Autodesk Inventor part; units mm, degrees
ref_plane "YZ Plane" through (0, 0, 0) normal (1, 0, 0) x (0, 1, 0)
ref_plane "XZ Plane" through (0, 0, 0) normal (0, 1, 0) x (-1, 0, 0)
ref_plane "XY Plane" through (0, 0, 0) normal (0, 0, 1) x (1, 0, 0)
sketch "Part" plane through (0, 0, 0) normal (1, 0, 0) x (0, 1, 0)
  line L0 (-0.5368, 0.0583) -> (59.7882, 0.0583) construction
  line L1 (-0.5371, -0.7417) -> (44.8022, -0.7417) construction
  arc A0 (59.7829, -0.7417) -> (59.7882, 0.0583) centre (-0.5368, 0.0583) ccw construction
  line L2 (-0.5368, 0.0583) -> (49.9741, -29.1042) construction
  arc A1 (47.3067, -27.5642) -> (54.7024, -0.7417) centre (-0.5368, 0.0583) ccw construction
  line L3 (69.9104, -5.8217) -> (54.3944, -5.8217) construction
  arc A2 (51.7936, -29.9522) -> (59.7829, -0.7417) centre (-0.5368, 0.0583) ccw construction
  line L4 (-0.5368, 0.0583) -> (66.9803, -116.8847) construction
  arc A3 (29.6257, -52.1846) -> (51.7936, -29.9522) centre (-0.5368, 0.0583) ccw
  arc A4 (27.0857, -47.7852) -> (54.3944, -5.8217) centre (-0.5368, 0.0583) ccw
  arc A5 (54.7024, -0.7417) -> (54.7082, 0.0583) centre (-0.5368, 0.0583) ccw construction
  line L5 (54.7024, -0.7417) -> (59.7829, -0.7417) construction
  line L6 (57.491, -5.8217) -> (54.3944, -5.8217) construction
  line L7 (44.8022, 0.0583) -> (44.8022, -0.7417) construction
  line L8 (44.8022, -0.7417) -> (44.8022, -5.8217)
  line L9 (44.8022, -5.8217) -> (44.8022, -11.0315) construction
  line L10 (44.8022, -0.7417) -> (57.7827, -0.7417)
  line L11 (44.8022, -5.8217) -> (-19.8971, -5.8217) construction
  line L12 (49.2882, 5.599) -> (49.2882, -56.7812) construction
  arc A6 (28.6257, -50.4526) -> (49.9741, -29.1042) centre (-0.5368, 0.0583) ccw construction
  line L13 (54.3944, -5.8217) -> (50.4651, -5.8217) construction
  line L14 (54.3944, -5.8217) -> (44.8022, -5.8217)
  line L15 (49.9741, -29.1042) -> (51.7936, -29.9522)
  arc A7 (49.9741, -29.1042) -> (57.7827, -0.7417) centre (-0.5368, 0.0583) ccw
  arc A8 (57.7827, -0.7417) -> (57.7882, 0.0583) centre (-0.5368, 0.0583) ccw construction
  line L16 (-0.5368, 0.0583) -> (-30.6993, -52.1846) construction
  line L17 (0.1561, -0.3414) -> (-22.5135, -39.6064) construction
  arc A9 (-30.6993, -52.1846) -> (-30.0039, -52.5801) centre (-0.5368, 0.0583) ccw construction
  line L18 (-0.5368, 0.0583) -> (-0.5368, -58.2667) construction
  arc A10 (-27.4636, -48.1802) -> (-0.5368, -55.1867) centre (-0.5368, 0.0583) ccw construction
  line L19 (-30.6682, -63.8907) -> (-22.9102, -50.4535) construction
  arc A11 (-30.0039, -52.5801) -> (-0.7122, -60.2664) centre (-0.5368, 0.0583) ccw construction
  arc A12 (-0.7122, -60.2664) -> (29.6257, -52.1846) centre (-0.5368, 0.0583) ccw
  arc A13 (-22.9102, -50.4535) -> (27.0857, -47.7852) centre (-0.5368, 0.0583) ccw
  arc A14 (-28.1593, -47.7852) -> (-27.4636, -48.1802) centre (-0.5368, 0.0583) ccw construction
  line L20 (-27.4636, -48.1802) -> (-30.0039, -52.5801) construction
  line L21 (-24.4585, -53.1353) -> (-22.9102, -50.4535) construction
  line L22 (-23.2063, -39.2064) -> (-22.5135, -39.6064) construction
  line L23 (-22.5135, -39.6064) -> (-18.1141, -42.1464)
  line L24 (-18.1141, -42.1464) -> (-13.6022, -44.7513) construction
  line L25 (-22.5135, -39.6064) -> (-29.0038, -50.8478)
  line L26 (-18.1141, -42.1464) -> (14.2355, 13.8848) construction
  line L27 (-30.2477, -40.3211) -> (23.7751, -71.5111) construction
  arc A15 (-0.5368, -58.2667) -> (28.6257, -50.4526) centre (-0.5368, 0.0583) ccw construction
  line L28 (-22.9102, -50.4535) -> (-20.9456, -47.0506) construction
  line L29 (-22.9102, -50.4535) -> (-18.1141, -42.1464)
  line L30 (-0.5368, -58.2667) -> (-0.7122, -60.2664)
  arc A16 (-29.0038, -50.8478) -> (-0.5368, -58.2667) centre (-0.5368, 0.0583) ccw
  arc A17 (-29.6993, -50.4526) -> (-29.0038, -50.8478) centre (-0.5368, 0.0583) ccw construction
  dimension "d29" = 60.325
  dimension "d32" = 30
  dimension "d35" = 5.08
  dimension "d37" = 60
  dimension "d38" = 55.245
  dimension "d42" = 14.986
  dimension "d44" = 10.5
  dimension "d45" = 58.325
  dimension "d64" = 0.8
extrude "Extrusion2" add sketch "Part" along normal blind 5.08
sketch "Sketch5" plane through (0, 44.8022, -0.7417) normal (0, 0, 1) x (1, 0, 0)
  line L0 (0, 12.9805) -> (5.08, 12.9805)
  line L1 (2.54, 12.9805) -> (2.54, 0) construction
  line L2 (0, 0) -> (5.08, 0)
  line L3 (0, 4.4805) -> (5.08, 4.4805) construction
  point P0 (0, -44.8022)
  point P1 (2.54, 4.4805)
  dimension "d48" = 8.5
hole "Hole1" at (2.54, 49.2827, -0.7417) direction (0, 0, -1) diameter 2.4384 depth 12.2936 tip angle 118
sketch "Sketch6" plane through (0, -29.0038, -50.8478) normal (0, -0.866, 0.5) x (1, 0, 0)
  line L0 (0, 12.9805) -> (5.08, 12.9805) construction
  line L1 (2.54, 12.9805) -> (2.54, 0) construction
  line L2 (0, 0) -> (5.08, 0) construction
  line L3 (0, 5.9891) -> (0, 58.4948) construction
  line L4 (0, 8.5) -> (5.08, 8.5) construction
  line L5 (5.08, 5.9891) -> (5.08, 58.4948) construction
  point P0 (0, 58.5374)
  point P1 (2.54, 8.5)
  dimension "d56" = 8.5
hole "Hole2" at (2.54, -24.7538, -43.4866) direction (0, 0.866, -0.5) diameter 2.4384 depth 12.2936 tip angle 118
equation "\"d35\" = d29 - d34"
properties part number "new_insert"
Geometry check sheet. Reference: the model listing, model coordinates, mm. A direction names the side the tool comes from. Round coordinates to 2 decimals unless told otherwise and drop trailing zeros. Loops run counter-clockwise (first coordinate to the right, second up) from the corner with the lowest first, then second, coordinate; pieces in that order, holes last. Notation, with made-up numbers: (19, 89.5) - (29, 89.5) arc R24 cw to (29, 115.5) - close; hole circle Ø7 at (-20, 17.5). An arc over 180 degrees is marked (long way). Use a Markdown table: item, result.
Q1. Cross-section at B-B on y = 19.5. Record the cut outline in (x, z).
Solutions:
| item | result |
|---|---|
| outline | (0, -56.84) - (5.08, -56.84) - (5.08, -51.43) - (0, -51.43) - close |
Q2. Cross-section at C-C on z = -24. Record the cut outline in (x, y).
Solutions:
| item | result |
|---|---|
| outline | (0, 49.19) - (5.08, 49.19) - (5.08, 52.6) - (0, 52.6) - close |
Q3. Cross-section at A-A on x = 2.54. Record the cut outline in (y, z), plus the area to 3 significant figures.
Solutions:
| item | result |
|---|---|
| outline | (-29, -50.85) arc R58.33 ccw to (-0.54, -58.27) - (-0.71, -60.27) arc R60.32 ccw to (29.63, -52.18) arc R60.33 ccw to (51.79, -29.95) - (49.97, -29.1) arc R58.33 ccw to (57.78, -0.74) - (50.5, -0.74) - (50.5, -5.82) - (54.39, -5.82) arc R55.25 cw to (27.09, -47.79) arc R55.24 cw to (-22.91, -50.45) - (-20.96, -47.08) - (-25.36, -44.54) - close; (-24.14, -42.43) - (-19.74, -44.97) - (-18.11, -42.15) - (-22.51, -39.61) - close; (44.8, -5.82) - (48.06, -5.82) - (48.06, -0.74) - (44.8, -0.74) - close |
| area | 561 mm2 |
Q4. Access from +Z, -Z, +X, -X, +Y, -Y to the whole of each face (thin tool, end or side, straight path). Record for faces 1 (the flat face through (2.5, 50.87, -29.52)), 2 (the cylindrical face through (2.504, 45.964, -29.769)), 3 (the flat face through (2.504, -0.623, -59.253)).
Solutions:
| item | result |
|---|---|
| face 1 | +X, -X, +Y |
| face 2 | +X, -X |
| face 3 | +X, -X, -Y |
Q5. Go/stop test with flat-tipped pins: P1, Ø1, axis at x = 3, y = 28.5, coming from the +Z side; P2, Ø3, axis at x = 2.54, y = 49.28, coming from the -Z side; P3, Ø3, axis at x = 1, z = -8.5, coming from the +Y side. Record where each tip stops, or that it passes through.
Solutions:
| item | result |
|---|---|
| P1 | stops at z = -46.63 |
| P2 | stops at z = -36.06 |
| P3 | stops at y = 57.36 |
Q6. Material ranges on line 1 (Z direction, x = 3.3, y = -22); line 2 (Z direction, x = 4.05, y = 50.5); line 3 (Y direction, x = 2.54, z = -3.1), recorded low to high.
Solutions:
| item | result |
|---|---|
| line 1 | z = -54.17 to -50.85, -48.88 to -46.18, -43.98 to -39.9 |
| line 2 | z = -32.1 to -29.35, -28.17 to -21.09, -5.82 to -0.74 |
| line 3 | y = 44.8 to 48.06, 50.5 to 57.7 |
Q7. Draft check along X on faces 4 (the flat face through (0, 27.04, -48)), 5 (the cylindrical face through (3.007, 48.156, -3.317)), 6 (the flat face through (2.5, -21.08, -47.28)), 7 (the flat face through (5.08, 27.04, -48)). Enter one of: released by +X, released by -X, zero draft, split by the parting line, or undercut.
Solutions:
| item | result |
|---|---|
| face 4 | released by -X |
| face 5 | undercut |
| face 6 | zero draft |
| face 7 | released by +X |
